```python
from build123d import *

# Parameters (mm, degrees)
BOSS_EXTRUDE1_START     = -4.7625
BOSS_EXTRUDE1_DEPTH     = 9.525
SKETCH4_R               = 3.175
CUT_EXTRUDE1_DEPTH      = 3.556
SKETCH5_R               = 1.778
CUT_EXTRUDE2_DEPTH      = 3.556
SKETCH6_R               = 1.778
CUT_EXTRUDE3_DEPTH      = 389.542033304
CUT_EXTRUDE4_DEPTH      = 3.556
CUT_EXTRUDE4_DEPTH_BACK = 388.321146479
SKETCH7_R               = 3.175
SKETCH7_R_2             = 1.778


# Read off the part's stored shape, not the designer's step: Boss-Extrude1
with BuildPart() as part:
    # Boss-Extrude1 outline → Boss-Extrude1 (new body)
    with BuildSketch(Plane(origin=(-0.151105159, 1.836314253, 0), x_dir=(-0.9999999911893379, -0.00013274533532885028, 0), z_dir=(0, 0, -1)).offset(BOSS_EXTRUDE1_START)):
        with BuildLine():
            add(Edge.make_bspline(
                [(266.719101765, -62.051598198), (285.372886056, -63.687772151), (308.740732669, -65.369335536), (332.113756278, -66.591725825), (336.786834388, -66.817774574)],
                knots=[0, 0, 0, 0, 0.444589519, 0.555671616, 0.555671616, 0.555671616, 0.555671616], degree=3))
            ThreePointArc((336.786834388, -66.817774574), (346.821832777, -65.271443631), (355.449407296, -59.918193219))
            Line((355.449407296, -59.918193219), (365.162167793, -50.749897782))
            Line((365.162167793, -50.749897782), (365.162167793, -42.440188824))
            ThreePointArc((365.162167793, -42.440188824), (366.092103763, -40.195124794), (368.337167793, -39.265188824))
            Line((368.337167793, -39.265188824), (377.328903503, -39.265188824))
            Line((377.328903503, -39.265188824), (383.403102119, -33.531489588))
            add(Edge.make_bspline(
                [(362.097911235, -32.917120768), (369.197743206, -33.164912437), (376.299473684, -33.369697882), (383.403102119, -33.531489588)],
                knots=[0.746516847, 0.746516847, 0.746516847, 0.746516847, 0.918535276, 0.918535276, 0.918535276, 0.918535276], degree=3))
            ThreePointArc((362.097911235, -32.917120768), (359.781604988, -33.806306666), (358.812167793, -36.090188824))
            Line((358.812167793, -36.090188824), (358.812167793, -45.273612359))
            ThreePointArc((358.812167793, -45.273612359), (358.293167277, -47.787960192), (356.821004007, -49.891300836))
            Line((356.821004007, -49.891300836), (351.090571083, -55.300504742))
            ThreePointArc((351.090571083, -55.300504742), (344.645600305, -59.305916448), (337.148417456, -60.4777614))
            add(Edge.make_bspline(
                [(302.92001028, -58.493795672), (304.509330321, -58.60122978), (315.913868956, -59.356827875), (327.324554644, -60.002877801), (337.148417456, -60.4777614)],
                knots=[0.283817359, 0.283817359, 0.283817359, 0.283817359, 0.321763123, 0.556088201, 0.556088201, 0.556088201, 0.556088201], degree=3))
            ThreePointArc((302.92001028, -58.493795672), (298.540134178, -56.306049329), (297.01844307, -51.652662937))
            ThreePointArc((297.01844307, -51.652662937), (298.817944258, -42.742557946), (302.676848033, -34.512306606))
            ThreePointArc((302.676848033, -34.512306606), (302.812285866, -31.389489502), (300.205974442, -29.663954561))
            add(Edge.make_bspline(
                [(290.723349608, -28.971987248), (293.88384664, -29.211203734), (297.044721601, -29.441859136), (300.205974442, -29.663954561)],
                knots=[0.169565869, 0.169565869, 0.169565869, 0.169565869, 0.246277706, 0.246277706, 0.246277706, 0.246277706], degree=3))
            ThreePointArc((290.723349608, -28.971987248), (287.894150829, -30.300881632), (287.574810624, -33.410278334))
            ThreePointArc((287.574810624, -33.410278334), (290.198038966, -42.113548005), (290.684983891, -51.190503181))
            ThreePointArc((290.684983891, -51.190503181), (288.503875799, -55.573685628), (283.852803221, -57.102425178))
            add(Edge.make_bspline(
                [(274.852701957, -56.374410111), (275.484326416, -56.427106964), (276.92498218, -56.546530571), (279.175001885, -56.730301658), (281.5434013, -56.92049496), (283.102708442, -57.04365577), (283.852803221, -57.102425178)],
                knots=[0.060364421, 0.060364421, 0.060364421, 0.060364421, 0.075455527, 0.094786271, 0.114117015, 0.132034547, 0.132034547, 0.132034547, 0.132034547], degree=3))
            Line((274.852701957, -56.374410111), (274.587380233, -59.554556157))
            Line((274.587380233, -59.554556157), (266.996524483, -58.888741635))
            Line((266.996524483, -58.888741635), (266.719101765, -62.051598198))
        make_face()
    extrude(amount=BOSS_EXTRUDE1_DEPTH)

    # Sketch4 → Cut-Extrude1 (cut)
    with BuildSketch(Plane(origin=(0.004968506, -37.428854199, 0), x_dir=(-0.999999991182225, -0.00013274533532793586, -3.771739900033909e-06), z_dir=(0.00013274533532888006, -0.999999991189338, 0))):
        with Locations(Location((373.034764896, -0.001423755, 0), (0, 0, 179.999783895))):
            Circle(SKETCH4_R)
    extrude(amount=-CUT_EXTRUDE1_DEPTH, mode=Mode.SUBTRACT)

    # Sketch5 → Cut-Extrude2 (cut)
    with BuildSketch(Plane(origin=(0.004496463, -33.872854231, 0), x_dir=(-0.999999991182225, -0.00013274533532793586, -3.771739900033909e-06), z_dir=(0.00013274533532888006, -0.9999999911893379, 0))):
        with Locations(Location((373.034764896, -0.001423755, 0), (0, 0, 179.999783895))):
            Circle(SKETCH5_R)
    extrude(amount=-CUT_EXTRUDE2_DEPTH, mode=Mode.SUBTRACT)

    # Sketch6 → Cut-Extrude3 (cut, through all)
    with BuildSketch(Plane(origin=(0.429757188, -5.878582453, 0), x_dir=(0.9973298035047504, 0.0729103752016881, 0.004164160074363476), z_dir=(-0.07291100735121511, 0.9973384505808602, 0))):
        with Locations(Location((-296.848920319, -1.255850637, 0), (0, 0, 180.238589487))):
            Circle(SKETCH6_R)
    extrude(amount=-CUT_EXTRUDE3_DEPTH, mode=Mode.SUBTRACT)

    # Sketch7 → Cut-Extrude4 (cut, two sides: drawn at the far end of the back side and taken through both)
    with BuildSketch(Plane(origin=(2.97617412, -40.71062784, 0), x_dir=(0.9973298035047504, 0.0729103752016881, 0.004164160074363476), z_dir=(-0.07291100735121511, 0.9973384505808603, 0)).offset(-CUT_EXTRUDE4_DEPTH_BACK)):
        with Locations(Location((-296.848920319, -1.255850637, 0), (0, 0, 180.238589487))):
            Circle(SKETCH7_R)
        with Locations(Location((-296.848920319, -1.255850637, 0), (0, 0, 180.238589487))):
            Circle(SKETCH7_R_2, mode=Mode.SUBTRACT)
    extrude(amount=CUT_EXTRUDE4_DEPTH + CUT_EXTRUDE4_DEPTH_BACK, mode=Mode.SUBTRACT)


solid = part.part
```
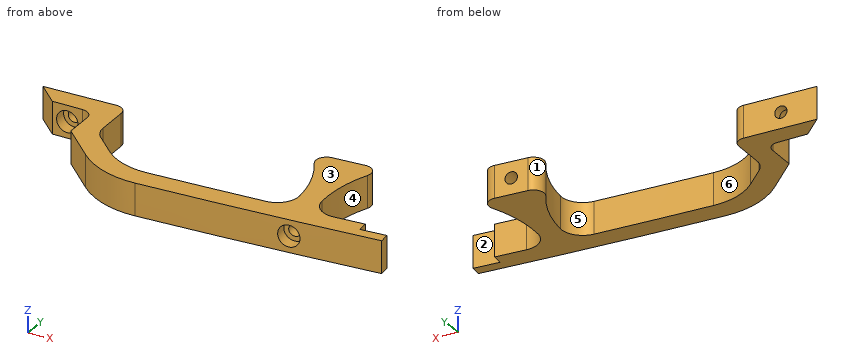
Design review of the part built by this model. Coordinates are the model's own, in mm. Face numbers are marked on the shaded views. A direction names the side the tool comes from. Coordinates: 2 decimals unless noted, no trailing zeros. Order: outer loops, then holes, each group sorted by start corner. A loop starts at its lowest first (then second) coordinate and runs counter-clockwise, first axis right, second up. Notation, with made-up numbers: (-9.5, 55.5) - (15.5, 55.5) arc R22 ccw to (15.5, 82.5) - close; hole circle Ø11 at (7.5, 6.5). An arc over 180 degrees is marked (long way). Answer in a Markdown table with one row per item.
(1) Consider section B-B on x = -342.5. State the section outline as (y, z) points.
Checked values:
| item | result |
|---|---|
| outline | (-64.68, -4.76) - (-58.2, -4.76) - (-58.2, 4.76) - (-64.68, 4.76) - close |
(2) The part is to be moulded in two halves that separate along Y. For the marked faces 1, 2 and 3, say which applies: released by +Y, released by -Y, zero draft, split by the parting line, or undercut.
Checked values:
| item | result |
|---|---|
| face 1 | undercut |
| face 2 | released by +Y |
| face 3 | zero draft |
(3) Consider section A-A on y = -45. Give the number of separate pieces and of enclosed holes in the cut face, plus the area to 3 significant figures.
Checked values:
| item | result |
|---|---|
| separate pieces | 2 |
| enclosed holes | 1 |
| area | 119 mm^2 |
(4) For the marked faces 4, 5 and 6, list the 3-axis set-ups (+Z, -Z, +X, -X, +Y, -Y) from which the entire face can be reached by the end or side of a thin tool; tool diameter is ignored.
Checked values:
| item | result |
|---|---|
| face 4 | +Z, -Z, +X |
| face 5 | +Z, -Z |
| face 6 | +Z, -Z, +Y |
(5) Clearance check with flat-ended pins moving along their axes: pin 1 (1.5 mm diameter, centred on y = -37.5, z = 1.5, fed in from -X); pin 2 (1 mm diameter, centred on y = -59.5, z = 1.5, fed in from -X); pin 3 (4 mm diameter, centred on x = -317.5, z = -1.5, fed in from -Y); pin 4 (12 mm diameter, centred on x = -280.5, y = -47, fed in from -Z). State where each tip first meets the part, or that it passes through.
Checked values:
| item | result |
|---|---|
| pin 1 | x = -378.25 |
| pin 2 | x = -354.62 |
| pin 3 | y = -64.1 |
| pin 4 | through |
(6) Wall thickness on line 1 along X through (y, z) = (-34.5, -2.25); line 2 along X through (y, z) = (-35.5, -2.25); line 3 along X through (y, z) = (-46, -3.5): over which ranges is each line inside the solid? List them lowest first. Write a range as from..to.
Checked values:
| item | result |
|---|---|
| line 1 | -380.63..-375.27, -370.79..-358.96, -301.78..-288.85 |
| line 2 | -379.57..-375.27, -370.79..-358.96, -301.24..-289.17 |
| line 3 | -365.31..-358.44, -297.67..-290.9 |
